Can you work these out from the model? Positions are in its coordinate system, mm. A direction names the side the tool comes from. Coordinates: 2 decimals unless noted, no trailing zeros. Loops run counter-clockwise (first coordinate to the right, second up) from the corner with the lowest first, then second, coordinate; pieces in that order, holes last.
```python
from build123d import *

# Parameters (mm, degrees)
SKETCH2_R          = 6.25
CUT_EXTRUDE1_DEPTH = 109.92456105


with BuildPart() as part:
    # Sketch1 → Revolve1 (revolve)
    with BuildSketch(Plane(origin=(0, 0, 0), x_dir=(1, 0, 0), z_dir=(0, 1, 0)), mode=Mode.PRIVATE) as revolve1_sk:
        Polygon((-44.2, 25), (-14.4, 25), (-14.4, 20), (29.8, 20), (29.8, 45), (44.2, 45), (44.2, 15), (20.4, 15), (-20.4, 15), (-20.2, 19), (-44.2, 19), align=None)
    revolve(revolve1_sk.sketch.rotate(Axis((-44.2, 0, 0), (1, 0, 0)), 180), axis=Axis((-44.2, 0, 0), (1, 0, 0)))

    # Sketch2 → Cut-Extrude1 (cut, through all)
    with BuildSketch(Plane(origin=(44.2, 0, 0), x_dir=(0, 0, -1), z_dir=(1, 0, 0))):
        with Locations((0, 32.5)):
            Circle(SKETCH2_R)
        with Locations((32.5, 0)):
            Circle(SKETCH2_R)
        with Locations((0, -32.5)):
            Circle(SKETCH2_R)
        with Locations((-32.5, 0)):
            Circle(SKETCH2_R)
    extrude(amount=-CUT_EXTRUDE1_DEPTH, mode=Mode.SUBTRACT)


solid = part.part
```
(1) I want a section at C-C on z = 35.5. Write out the boundary of the cut face in (x, y).
Check values:
outline: (29.8, -27.65) - (44.2, -27.65) - (44.2, -5.48) - (29.8, -5.48) - close; (29.8, 5.48) - (44.2, 5.48) - (44.2, 27.65) - (29.8, 27.65) - close
(2) I want a section at A-A on z = 0. Write out the boundary of the cut face in (x, y).
Check values:
outline: (-44.2, -25) - (-14.4, -25) - (-14.4, -20) - (29.8, -20) - (29.8, -26.25) - (44.2, -26.25) - (44.2, -15) - (-20.4, -15) - (-20.2, -19) - (-44.2, -19) - close; (-44.2, 19) - (-20.2, 19) - (-20.4, 15) - (44.2, 15) - (44.2, 26.25) - (29.8, 26.25) - (29.8, 20) - (-14.4, 20) - (-14.4, 25) - (-44.2, 25) - close; (29.8, -45) - (44.2, -45) - (44.2, -38.75) - (29.8, -38.75) - close; (29.8, 38.75) - (44.2, 38.75) - (44.2, 45) - (29.8, 45) - close
(3) I'm going to push flat-ended pins straight in: pin 1 (10 mm diameter, centred on y = 32.5, z = 0, fed in from +X); pin 2 (6 mm diameter, centred on x = -7, z = -13, fed in from -Y); pin 3 (14.5 mm diameter, centred on y = 0, z = -32.5, fed in from +X); pin 4 (3 mm diameter, centred on x = -6.5, z = 0.5, fed in from -Y). Where does each tip first touch, or does it pass through?
Check values:
pin 1: passes through
pin 2: stops at y = -17.32
pin 3: stops at x = 44.2
pin 4: stops at y = -20
(4) If I drill on probe 1 along Y at (x, z) = (31.5, 0); probe 2 along X at (y, z) = (-20, 4); probe 3 along Y at (x, z) = (-28.5, 0), over which ranges is the centre line in solid material (lowest first)?
Check values:
probe 1: y = -45 to -38.75, -26.25 to -15, 15 to 26.25, 38.75 to 45
probe 2: x = -44.2 to -14.4, 29.8 to 44.2
probe 3: y = -25 to -19, 19 to 25
(5) Which directions (+Z, -Z, +X, -X, +Y, -Y) give clear straight access to the entire face, cutting with the end or side of a thin tool? Please do faces 4 (the cylindrical face through (-32.368, 18.548, -4.119)), 5 (the cylindrical face through (8.01, -0.88, -19.98)), 6 (the flat face through (-44.2, -19, 4)).
Check values:
face 4: -X
face 5: none
face 6: +Z, -Z, -X, +Y, -Y
(6) I want a section at B-B on y = 32.5. Write out the boundary of the cut face in (x, z), then the cut area to 3 significant figures.
Check values:
outline: (29.8, -31.12) - (44.2, -31.12) - (44.2, -6.25) - (29.8, -6.25) - close; (29.8, 6.25) - (44.2, 6.25) - (44.2, 31.12) - (29.8, 31.12) - close
area: 716 mm2
(7) If we mould it in two halves opening along Y, with no side actions, what happens to faces 1 (the cylindrical face through (37.1, -30.62, -5.96)), 2 (the cylindrical face through (37.101, 39.923, 20.765)), 3 (the flat face through (29.8, 19, -9))? For each: released by +Y, released by -Y, zero draft, split by the parting line, or undercut.
Check values:
face 1: undercut
face 2: split by the parting line
face 3: zero draft
(8) I want a section at D-D on x = 1. Write out the boundary of the cut face in (y, z), then the cut area to 3 significant figures.
Check values:
outline: circle Ø40 at (0, 0); hole circle Ø30 at (0, 0)
area: 550 mm2
